Autodesk Inventor part; units mm, degrees
ref_plane "YZ Plane" through (0, 0, 0) normal (1, 0, 0) x (0, 1, 0)
ref_plane "XZ Plane" through (0, 0, 0) normal (0, 1, 0) x (-1, 0, 0)
ref_plane "XY Plane" through (0, 0, 0) normal (0, 0, 1) x (1, 0, 0)
sketch "Sketch1" plane through (0, 0, 0) normal (0, 1, 0) x (-1, 0, 0)
  line L0 (0, 0) -> (-336, 0)
  line L1 (-336, 0) -> (-336, -15)
  line L2 (-336, -15) -> (0, -15)
  line L3 (0, -15) -> (0, 0)
  dimension "d0" = 15
  dimension "d1" = 336
extrude "Extrusion1" add sketch "Sketch1" along normal blind 6.5
sketch "Sketch2" plane through (0, 6.5, 0) normal (0, 1, 0) x (1, 0, 0)
  line L0 (0, 0) -> (336, 0)
  line L1 (336, 0) -> (336, 15)
  line L2 (0, 15) -> (0, 0)
  line L3 (0, 12) -> (-4.5, 12)
  line L4 (-6.5, 10) -> (-6.5, 6)
  line L5 (-4.5, 4) -> (0, 4)
  line L6 (0, 4) -> (0, 12)
  line L7 (336, 12) -> (340.5, 12)
  line L8 (342.5, 10) -> (342.5, 6)
  line L9 (340.5, 4) -> (336, 4)
  line L10 (336, 4) -> (336, 12)
  line L11 (80, 0) -> (88, 0)
  line L12 (88, 0) -> (88, -4.5)
  line L13 (86, -6.5) -> (82, -6.5)
  line L14 (80, -4.5) -> (80, 0)
  line L15 (248, 0) -> (256, 0)
  line L16 (256, 0) -> (256, -4.5)
  line L17 (254, -6.5) -> (250, -6.5)
  line L18 (248, -4.5) -> (248, 0)
  arc A0 (-4.5, 12) -> (-6.5, 10) centre (-4.5, 10) ccw
  arc A1 (-6.5, 6) -> (-4.5, 4) centre (-4.5, 6) ccw
  arc A2 (80, -4.5) -> (82, -6.5) centre (82, -4.5) ccw
  arc A3 (86, -6.5) -> (88, -4.5) centre (86, -4.5) ccw
  arc A4 (248, -4.5) -> (250, -6.5) centre (250, -4.5) ccw
  arc A5 (254, -6.5) -> (256, -4.5) centre (254, -4.5) ccw
  arc A6 (340.5, 4) -> (342.5, 6) centre (340.5, 6) ccw
  arc A7 (342.5, 10) -> (340.5, 12) centre (340.5, 10) ccw
  dimension "d4" = 2
  dimension "d5" = 8
  dimension "d6" = 8
  dimension "d7" = 8
  dimension "d8" = 8
  dimension "d9" = 6.5
  dimension "d10" = 6.5
  dimension "d11" = 6.5
  dimension "d12" = 4
  dimension "d13" = 80
  dimension "d14" = 80
extrude "Extrusion2" add sketch "Sketch2" against normal blind 6.5
equation "\"d6\" = d5"
equation "\"d7\" = d6"
equation "\"d8\" = d7"
equation "\"d10\" = d9"
equation "\"d11\" = d9"
equation "\"d14\" = d13"
properties part number "front_upper_brace" material "Plywood, Finish"
Input: part model. Units: mm. Frame: model coordinates. A direction names the side the tool comes from. Give positions to 0.01 mm unless a question says otherwise; leave off trailing zeros. Write each loop counter-clockwise with the first axis right and the second up, starting at its lowest first coordinate (ties: lowest second). Pieces come first, ordered by that corner, then holes. Notation, with made-up numbers: (8, 49) - (39, 49) arc R36 cw to (39, 87) - close; hole circle Ø10 at (-21.5, -10.5). An arc over 180 degrees is marked (long way). Write item = value, one per line. Start each with the question number.
1) Cut plane B-B (x = 197). Return loops of the section in (y, z), and give its area (3 significant figures).
2) Cut plane A-A (y = 5.5). Return loops of the section in (x, z).
3) Reachability of faces 1 (the face through (170, 3, -15)), 2 (the face through (167, 3, 0)), 3 (the face through (39, 3, 0)), 4 (the face through (295, 3, 0)) from +Z, -Z, +X, -X, +Y, -Y: full face, straight path, thin tool, end or side. Return the list, or none.
4) Pin query (flat end, axial travel): pin 1 (2 mm diameter, centred on x = -1.5, y = 3.5, fed in from +Z); pin 2 (1 mm diameter, centred on x = 275.5, y = 1.5, fed in from +Z); pin 3 (2 mm diameter, centred on y = 3.5, z = -2, fed in from +X). Return the tip coordinate at first contact, or that it passes through.
5) Material intervals for L1, parallel to X at y = 3.75, z = 3.5; L2, parallel to Z at x = 66, y = 2.5; L3, parallel to X at y = 2.75, z = -14, sorted ascending. Write a range as [from, to].
Answers follow:
q1.outline = (0, -15) - (6.5, -15) - (6.5, 0) - (0, 0) - close
q1.area = 97.5 mm^2
q2.outline = (-6.5, -10) arc R2 ccw to (-4.5, -12) - (0, -12) - (0, -15) - (336, -15) - (336, -12) - (340.5, -12) arc R2 ccw to (342.5, -10) - (342.5, -6) arc R2 ccw to (340.5, -4) - (336, -4) - (336, 0) - (256, 0) - (256, 4.5) arc R2 ccw to (254, 6.5) - (250, 6.5) arc R2 ccw to (248, 4.5) - (248, 0) - (88, 0) - (88, 4.5) arc R2 ccw to (86, 6.5) - (82, 6.5) arc R2 ccw to (80, 4.5) - (80, 0) - (0, 0) - (0, -4) - (-4.5, -4) arc R2 ccw to (-6.5, -6) - close
q3.face_1 = -Z, +X, -X, +Y, -Y
q3.face_2 = +Z, +Y, -Y
q3.face_3 = +Z, -X, +Y, -Y
q3.face_4 = +Z, +X, +Y, -Y
q4.pin_1 = -4
q4.pin_2 = 0
q4.pin_3 = 336
q5.L1 = [80, 88], [248, 256]
q5.L2 = [-15, 0]
q5.L3 = [0, 336]
